from build123d import *

# Parameters (mm, degrees)
SKETCH1_W           = 25.4
SKETCH1_H           = 27
SKETCH1_R           = 1.75
BOSS_EXTRUDE1_DEPTH = 3.175
SKETCH2_W           = 16.51
SKETCH2_H           = 6.35
CUT_EXTRUDE1_DEPTH  = 28
BOSS_EXTRUDE2_DEPTH = 27
SKETCH4_R           = 1.75
CUT_EXTRUDE2_DEPTH  = 13.7
SKETCH5_R           = 3
CUT_EXTRUDE3_DEPTH  = 6.35
FILLET1_R           = 2.54


with BuildPart() as part:
    # Sketch1 → Boss-Extrude1 (new body, symmetric)
    with BuildSketch(Plane(origin=(0, 0, 0), x_dir=(1, 0, 0), z_dir=(0, 1, 0))):
        Rectangle(SKETCH1_W, SKETCH1_H)
        with Locations((-10.16, 0)):
            Circle(SKETCH1_R, mode=Mode.SUBTRACT)
        with Locations((10.16, 0)):
            Circle(SKETCH1_R, mode=Mode.SUBTRACT)
    extrude(amount=BOSS_EXTRUDE1_DEPTH, both=True)

    # Sketch2 → Cut-Extrude1 (cut, through all)
    with BuildSketch(Plane.XY.offset(13.5)):
        Rectangle(SKETCH2_W, SKETCH2_H)
    extrude(amount=-CUT_EXTRUDE1_DEPTH, mode=Mode.SUBTRACT)

    # Sketch3 → Boss-Extrude2 (add, through all)
    with BuildSketch(Plane.XY.offset(13.5)):
        with BuildLine():
            Line((-12.7, 3.175), (-8.255, 3.175))
            ThreePointArc((-8.255, 3.175), (0, 11.557), (8.255, 3.175))
            Line((8.255, 3.175), (12.7, 3.175))
            ThreePointArc((12.7, 3.175), (0, 15.875), (-12.7, 3.175))
        make_face()
    extrude(amount=-BOSS_EXTRUDE2_DEPTH)

    # Sketch4 → Cut-Extrude2 (cut, through all)
    with BuildSketch(Plane.XZ.offset(-3.175)):
        with Locations((-10.16, 0)):
            Circle(SKETCH4_R)
        with Locations((10.16, 0)):
            Circle(SKETCH4_R)
    extrude(amount=-CUT_EXTRUDE2_DEPTH, mode=Mode.SUBTRACT)

    # Sketch5 → Cut-Extrude3 (cut)
    with BuildSketch(Plane(origin=(0, 15.875, 0), x_dir=(1, 0, 0), z_dir=(0, 1, 0))):
        with Locations((-10.16, 0)):
            Circle(SKETCH5_R)
        with Locations((10.16, 0)):
            Circle(SKETCH5_R)
    extrude(amount=-CUT_EXTRUDE3_DEPTH, mode=Mode.SUBTRACT)

    # Fillet1
    fillet1_edges = [part.edges().sort_by_distance(p)[0] for p in [
        (0, 15.875, -13.5),
        (0, 15.875, 13.5),
        (12.7, 0, -13.5),
        (12.7, 0, 13.5),
        (-12.7, 0, -13.5),
        (-12.7, 0, 13.5),
    ]]
    fillet(fillet1_edges, radius=FILLET1_R)


solid = part.part
Source: CAD feature listing. Evaluate the final solid. Frame: model axes, mm. A direction names the side the tool comes from. Round coordinates to 2 decimals unless told otherwise and drop trailing zeros. Loops run counter-clockwise (first coordinate to the right, second up) from the corner with the lowest first, then second, coordinate; pieces in that order, holes last. Notation, with made-up numbers: (-30, -24) - (-23, -24) arc R23 ccw to (-23, 4) - close; hole circle Ø6 at (-6, -21.5). An arc over 180 degrees is marked (long way). Write item = value, one per line. Start each with the question number.
Item 1: Section query A-A on z = -8. Output: boundary loops of the cut face in (x, y) (3 decimals), plus the area to 3 significant figures.
Item 2: Material intervals for line 1 (X direction, y = -0.75, z = 0) (3 decimals); line 2 (Z direction, x = -10.16, y = 1.75); line 3 (X direction, y = 6, z = 0), sorted ascending.
Item 3: Section query C-C on x = 0. Output: boundary loops of the cut face in (y, z) (3 decimals).
Item 4: Mould query, pull axis Z, two halves, no side actions, for faces 1 (the face through (0, 12, -13.5)), 2 (the face through (8, 9.525, 0)), 3 (the face through (11.976, 0.044, 12.736)). Classes: released by +Z, released by -Z, zero draft, split by the parting line, or undercut.
Item 5: Section query B-B on y = 7. Count the separate pieces of the cut face and the enclosed holes in it, plus the area to 3 significant figures.
Item 6: First-contact query: pin 1 Ø5.5 at (x, z) = (10.16, 0) entering from +Y (3 decimals); pin 2 Ø1.5 at (y, z) = (10.5, -3.5) entering from +X; pin 3 Ø1.5 at (x, z) = (1.5, -4.5) entering from +Y. Flat tips, straight axial feed; report the tip coordinate or a pass-through.
Item 7: Reachability of faces 4 (the face through (12.4, -3.175, -0.2)), 5 (the face through (-8.255, 0, 0)) from +Z, -Z, +X, -X, +Y, -Y: full face, straight path, thin tool, end or side. Return the list, or none.
Results list:
q1.outline = (-12.7, -3.175) - (-8.255, -3.175) - (-8.255, 3.175) arc R8.256 cw (long way) to (8.255, 3.175) - (8.255, -3.175) - (12.7, -3.175) - (12.7, 3.175) arc R12.7 ccw to (-12.7, 3.175) - close
q1.area = 201 mm²
q2.line_1 = -12.7 to -11.91, -8.41 to -8.255, 8.255 to 8.41, 11.91 to 12.7
q2.line_2 = -13.5 to -1.75, 1.75 to 13.5
q2.line_3 = -12.38 to -11.91, -8.41 to -7.8, 7.8 to 8.41, 11.91 to 12.38
q3.outline = (11.557, -13.5) - (13.335, -13.5) arc R2.54 ccw to (15.875, -10.96) - (15.875, 10.96) arc R2.54 ccw to (13.335, 13.5) - (11.557, 13.5) - close
q4.face_1 = released by -Z
q4.face_2 = undercut
q4.face_3 = released by +Z
q5.separate_pieces = 2
q5.enclosed_holes = 2
q5.area = 230 mm²
q6.pin_1 = 9.525
q6.pin_2 = 10.87
q6.pin_3 = 15.85
q7.face_4 = +Z, -Z, +X, -X, -Y
q7.face_5 = +Z, -Z, -Y
